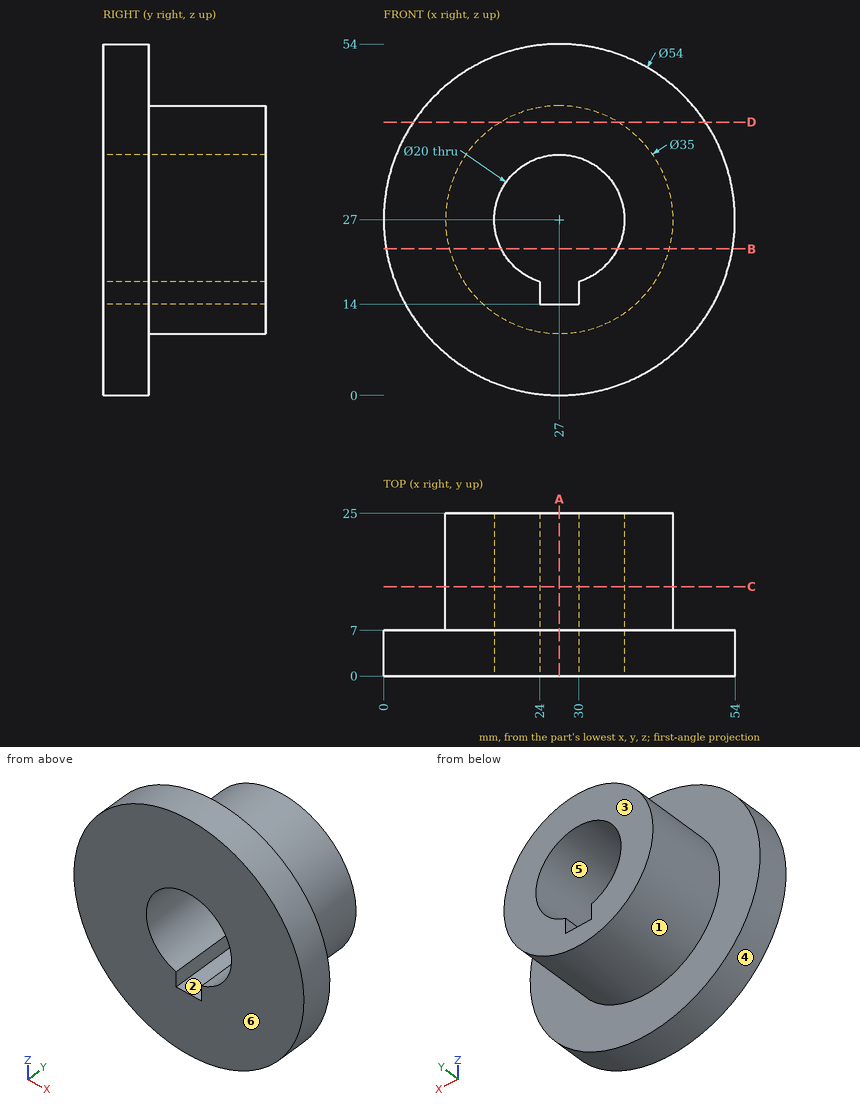
Study the drawing (mm; zero at the part's minimum x, y, z) and answer. A direction names the side the tool comes from. Coordinates: 2 decimals unless noted, no trailing zeros. Write each loop counter-clockwise with the first axis right and the second up, starting at its lowest first coordinate (ties: lowest second). Pieces come first, ordered by that corner, then holes. Notation, with made-up numbers: (65, -30.75) - (72, -30.75) arc R14 cw to (72, -3.75) - close; hole circle Ø10 at (-6, 73.25). An arc over 180 degrees is marked (long way). Return JSON: item names as keys, results as strings. Group by question number.
1. Given pin 1 (4 mm diameter, centred on y = 7, z = 15.5, fed in from +X); pin 2 (1.5 mm diameter, centred on x = 16, y = 5.5, fed in from -Z); pin 3 (2 mm diameter, centred on x = 46, y = 7, fed in from +Z), each flat-ended and moving along its own axis, determine where each tip first touches the part or whether it passes through.
2. A cutting plane is placed at D-D, the plane z = 42. Determine the outline of the cut face in (x, y), plus the area to 3 significant figures.
3. A cutting plane is placed at A-A, the plane x = 27. Determine the outline of the cut face in (y, z), plus the area to 3 significant figures.
4. Which of the six approach directions +Z, -Z, +X, -X, +Y, -Y give full straight-line access (tool end or side, diameter ignored) to the marked faces 1, 2 and 3?
5. A cutting plane is placed at B-B, the plane z = 22.5. Determine the outline of the cut face in (x, y).
6. Determine the mould class of the marked faces 4, 5 and 6 for opening direction X: released by +X, released by -X, zero draft, split by the parting line, or undercut.
7. A cutting plane is placed at C-C, the plane y = 13.75. Determine the outline of the cut face in (x, z), plus the area to 3 significant figures.
8. Straight lines are drawn through the part: L1, parallel to X at y = 8.5, z = 27; L2, parallel to Y at x = 20, z = 7; L3, parallel to X at y = 5.75, z = 15. For each, find the intervals that lie inside material, in ascending order.
Ans:
{
 "1": {"pin 1": "x = 52.27", "pin 2": "z = 2.02", "pin 3": "z = 47.12"},
 "2": {"outline": "(4.55, 0) - (49.45, 0) - (49.45, 7) - (36.01, 7) - (36.01, 25) - (17.99, 25) - (17.99, 7) - (4.55, 7) - close", "area": "639 mm²"},
 "3": {"outline": "(0, 0) - (7, 0) - (7, 9.5) - (25, 9.5) - (25, 14) - (0, 14) - close; (0, 37) - (25, 37) - (25, 44.5) - (7, 44.5) - (7, 54) - (0, 54) - close", "area": "433 mm²"},
 "4": {"face 1": "+Y", "face 2": "+Y, -Y", "face 3": "+Z, -Z, +X, -X, +Y"},
 "5": {"outline": "(0.38, 0) - (18.07, 0) - (18.07, 25) - (10.09, 25) - (10.09, 7) - (0.38, 7) - close; (35.93, 0) - (53.62, 0) - (53.62, 7) - (43.91, 7) - (43.91, 25) - (35.93, 25) - close"},
 "6": {"face 4": "split by the parting line", "face 5": "undercut", "face 6": "zero draft"},
 "7": {"outline": "circle Ø35 at (27, 27); hole (24, 14) - (30, 14) - (30, 17.46) arc R10 ccw (long way) to (24, 17.46) - close", "area": "629 mm²"},
 "8": {"L1": "9.5 to 17, 37 to 44.5", "L2": "0 to 7", "L3": "2.81 to 24, 30 to 51.19"}
}
